```python
from build123d import *

# Parameters (mm, degrees)
SKETCH1_W           = 200
SKETCH1_H           = 200
BOSS_EXTRUDE1_DEPTH = 10
SKETCH4_R           = 5
BOSS_EXTRUDE2_DEPTH = 100


with BuildPart() as part:
    # Sketch1 → Boss-Extrude1 (new body)
    with BuildSketch(Plane.XY):
        with Locations((100, 100)):
            Rectangle(SKETCH1_W, SKETCH1_H)
    extrude(amount=BOSS_EXTRUDE1_DEPTH)

    # Sketch4 → Boss-Extrude2 (add)
    with BuildSketch(Plane(origin=(0, 0, 0), x_dir=(-1, 0, 0), z_dir=(0, 0, -1))):
        with Locations((-190, 100)):
            Circle(SKETCH4_R)
        with Locations((-100, 10)):
            Circle(SKETCH4_R)
        with Locations((-100, 190)):
            Circle(SKETCH4_R)
        with Locations((-10, 100)):
            Circle(SKETCH4_R)
    extrude(amount=-BOSS_EXTRUDE2_DEPTH)


solid = part.part
```
The model under review builds one solid part; all positions refer to its coordinate system, in mm. A direction names the side the tool comes from. Coordinates: 2 decimals unless noted, no trailing zeros. Write each loop counter-clockwise with the first axis right and the second up, starting at its lowest first coordinate (ties: lowest second). Pieces come first, ordered by that corner, then holes. Notation, with made-up numbers: (89, 75.5) - (107, 75.5) arc R26 cw to (107, 95.5) - close; hole circle Ø1 at (16, 30.5). An arc over 180 degrees is marked (long way). Write item = value, one per line.
(1) Consider section B-B, the plane x = 190. Give the boundary of the cut face in (y, z).
Result sheet:
outline = (0, 0) - (200, 0) - (200, 10) - (105, 10) - (105, 100) - (95, 100) - (95, 10) - (0, 10) - close
(2) Consider section C-C, the plane z = 85.5. Give the boundary of the cut face in (x, y).
Result sheet:
outline = circle Ø10 at (10, 100); circle Ø10 at (100, 10); circle Ø10 at (100, 190); circle Ø10 at (190, 100)
(3) Mouldability with a two-part tool opening along Y and no side actions: class faces 3 (the face through (100.651, 194.957, 54.37)), 4 (the face through (99, 200, 5)), 5 (the face through (5.23, 101.5, 54.37)), 6 (the face through (190, 100, 100)) as pulls with the +Y half, pulls with the -Y half, needs draft (parallel to the pull), parting line crosses it, or undercut.
Result sheet:
face_3 = undercut
face_4 = pulls with the +Y half
face_5 = parting line crosses it
face_6 = needs draft
(4) Consider section D-D, the plane x = 109. Give the boundary of the cut face in (y, z).
Result sheet:
outline = (0, 0) - (200, 0) - (200, 10) - (0, 10) - close
(5) Machinability: for faces 1 (the face through (195, 100, 54)), 2 (the face through (100, 10, 100)), which of the approach directions +Z, -Z, +X, -X, +Y, -Y give a long, thin tool a straight path to every point of the face, cutting with its end or side? Answer none if there is none.
Result sheet:
face_1 = +Z
face_2 = +Z, +X, -X, +Y, -Y
(6) For line 1 (Z direction, x = 179, y = 173); line 2 (Y direction, x = 9, z = 59.5); line 3 (Y direction, x = 101, z = 20), list the stretches that pass through material, from the lowest coordinate up. Write a range as [from, to].
Result sheet:
line_1 = [0, 10]
line_2 = [95.1, 104.9]
line_3 = [5.1, 14.9], [185.1, 194.9]
(7) Consider section A-A, the plane y = 100. Give the boundary of the cut face in (x, z).
Result sheet:
outline = (0, 0) - (200, 0) - (200, 10) - (195, 10) - (195, 100) - (185, 100) - (185, 10) - (15, 10) - (15, 100) - (5, 100) - (5, 10) - (0, 10) - close
